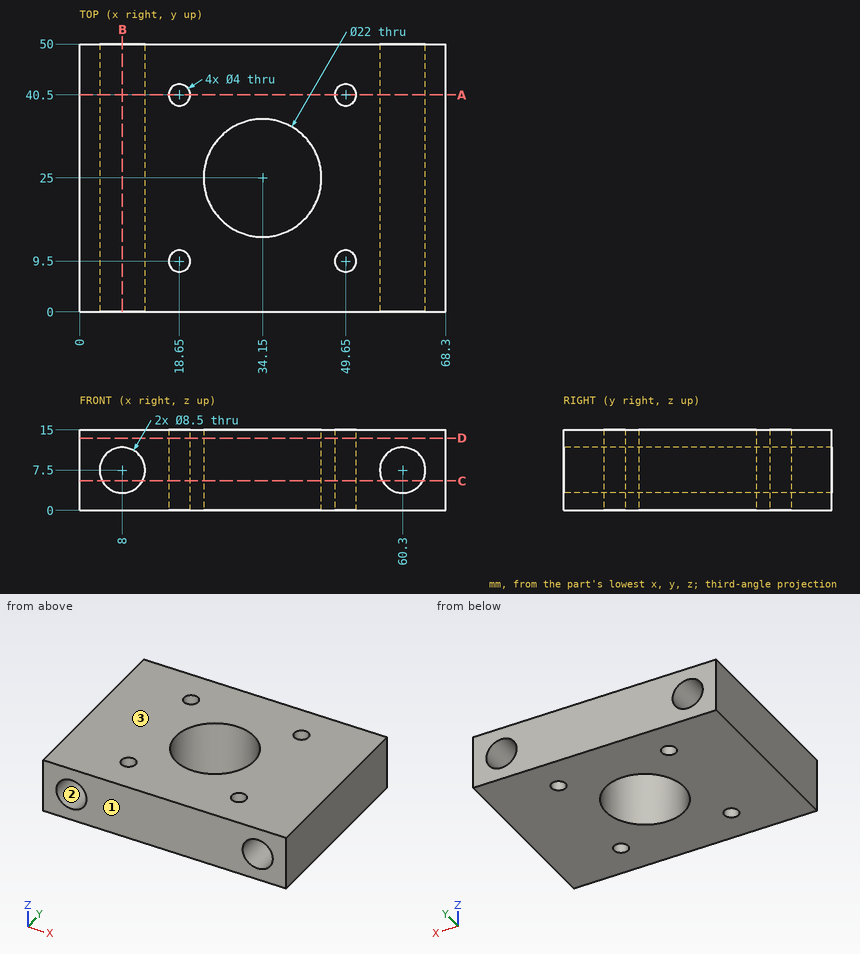
Geometry check sheet. Reference: drawing and pictorial views, mm from the part's lowest x, y, z. Give positions to 0.01 mm unless a question says otherwise; leave off trailing zeros. Write each loop counter-clockwise with the first axis right and the second up, starting at its lowest first coordinate (ties: lowest second). Pieces come first, ordered by that corner, then holes. Notation, with made-up numbers: M 76,28.5 L 80,28.5 A18 ccw 80,43.5 Z; hole C 75.5,21.25 d2. An arc over 180 degrees is marked long. Answer as CSV lines item,"result". Start each with the question number.
Q1. Material ranges on L1, parallel to X at y = 21.5, z = 3.75; L2, parallel to X at y = 29, z = 6.25; L3, parallel to Y at x = 48, z = 3.5, recorded low to high.
Q2. Release check for a two-part mould opening along Z. For the marked faces 1, 2 and 3 record: pulls with the +Z half, pulls with the -Z half, needs draft (parallel to the pull), parting line crosses it, or undercut.
Q3. Section check C-C, the plane z = 5.5. Record the cut outline in (x, y).
Q4. Section check B-B, the plane x = 8. Record the cut outline in (y, z).
Q5. Section check D-D, the plane z = 13.5. Record the cut outline in (x, y), then the cut area to 3 significant figures.
Q6. Section check A-A, the plane y = 40.5. Record the cut outline in (x, z), then the cut area to 3 significant figures.
Geometry says:
1,L1,"0 to 6, 10 to 23.72, 44.58 to 58.3, 62.3 to 68.3"
1,L2,"0 to 3.94, 12.06 to 23.9, 44.4 to 56.24, 64.36 to 68.3"
1,L3,"0 to 8.37, 10.63 to 39.37, 41.63 to 50"
2,face 1,"needs draft"
2,face 2,"undercut"
2,face 3,"pulls with the +Z half"
3,outline,"M 0,0 L 4.25,0 L 4.25,50 L 0,50 Z; M 11.75,0 L 56.55,0 L 56.55,50 L 11.75,50 Z; M 64.05,0 L 68.3,0 L 68.3,50 L 64.05,50 Z; hole C 18.65,9.5 d4; hole C 18.65,40.5 d4; hole C 34.15,25 d22; hole C 49.65,9.5 d4; hole C 49.65,40.5 d4"
4,outline,"M 0,0 L 50,0 L 50,3.25 L 0,3.25 Z; M 0,11.75 L 50,11.75 L 50,15 L 0,15 Z"
5,outline,"M 0,0 L 68.3,0 L 68.3,50 L 0,50 Z; hole C 18.65,9.5 d4; hole C 18.65,40.5 d4; hole C 34.15,25 d22; hole C 49.65,9.5 d4; hole C 49.65,40.5 d4"
5,area,"2,980 mm^2"
6,outline,"M 0,0 L 16.65,0 L 16.65,15 L 0,15 Z; M 20.65,0 L 47.65,0 L 47.65,15 L 20.65,15 Z; M 51.65,0 L 68.3,0 L 68.3,15 L 51.65,15 Z; hole C 8,7.5 d8.5; hole C 60.3,7.5 d8.5"
6,area,"791 mm^2"
